Geometry: final body of the model. Coordinates: model frame, mm. A direction names the side the tool comes from. Round coordinates to 2 decimals unless told otherwise and drop trailing zeros. Answer in a Markdown table with one row per item.
Autodesk Inventor part; units mm, degrees
ref_plane "YZ Plane" through (0, 0, 0) normal (1, 0, 0) x (0, 1, 0)
ref_plane "XZ Plane" through (0, 0, 0) normal (0, 1, 0) x (-1, 0, 0)
ref_plane "XY Plane" through (0, 0, 0) normal (0, 0, 1) x (1, 0, 0)
sketch "Sketch1" plane through (0, 0, 0) normal (0, 0, 1) x (1, 0, 0)
  line L0 (-228.6, 101.6) -> (228.6, 101.6)
  line L1 (228.6, 101.6) -> (228.6, -101.6)
  line L2 (228.6, -101.6) -> (-228.6, -101.6)
  line L3 (-228.6, -101.6) -> (-228.6, 101.6)
  point P0 (0, 0)
  dimension "d0" = 457.2
  dimension "d1" = 203.2
  dimension "d2" = 228.6
  dimension "d3" = 101.6
extrude "Extrusion1" add sketch "Sketch1" along normal blind 6.35
sketch "Sketch2" plane through (0, 0, 6.35) normal (0, 0, 1) x (1, 0, 0)
  line L0 (-228.6, -101.6) -> (228.6, -101.6)
  line L1 (-196.85, -101.6) -> (-158.75, -101.6)
  line L2 (-158.75, -101.6) -> (-158.75, -63.5)
  line L3 (-158.75, -63.5) -> (-196.85, -63.5)
  line L4 (-196.85, -63.5) -> (-196.85, -101.6)
  line L5 (158.75, -101.6) -> (196.85, -101.6)
  line L6 (196.85, -101.6) -> (196.85, -63.5)
  line L7 (196.85, -63.5) -> (158.75, -63.5)
  line L8 (158.75, -63.5) -> (158.75, -101.6)
  line L9 (-228.6, 101.6) -> (-228.6, -101.6)
  line L10 (228.6, -101.6) -> (228.6, 101.6)
  point P0 (0, 0)
  dimension "d6" = 31.75
  dimension "d7" = 38.1
  dimension "d8" = 38.1
  dimension "d9" = 31.75
extrude "Extrusion2" cut sketch "Sketch2" against normal through all
chamfer "Chamfer1" distance 6.35 angle 45 4 edges at (196.85, -101.6, 3.175) (158.75, -101.6, 3.175) (-196.85, -101.6, 3.175) (-158.75, -101.6, 3.175)
sketch "Sketch3" plane through (0, 0, 0) normal (0, 0, -1) x (-1, 0, 0)
  circle A0 centre (-209.55, -88.9) radius 3.175
  circle A1 centre (-146.05, -88.9) radius 3.175
  circle A2 centre (146.05, -88.9) radius 3.175
  circle A3 centre (209.55, -88.9) radius 3.175
  line L0 (-152.4, -101.6) -> (152.4, -101.6)
  line L1 (-228.6, 101.6) -> (-228.6, -101.6)
  line L2 (228.6, -101.6) -> (228.6, 101.6)
  point P0 (0, 0)
  dimension "d15" = 12.7
  dimension "d16" = 6.35
  dimension "d17" = 19.05
  dimension "d18" = 63.5
  dimension "d19" = 63.5
  dimension "d20" = 19.05
extrude "Extrusion3" cut sketch "Sketch3" against normal blind 25.4
sketch "Sketch4" plane through (0, 0, 0) normal (0, 0, -1) x (-1, 0, 0)
  circle A0 centre (139.7, 76.2) radius 3.302
  circle A1 centre (165.1, 88.9) radius 3.302
  circle A2 centre (190.5, 76.2) radius 3.302
  circle A3 centre (215.9, 88.9) radius 3.302
  circle A4 centre (147.0661, 22.2869) radius 2.513
  circle A5 centre (177.1772, 22.2869) radius 2.513
  circle A6 centre (207.2882, 22.2869) radius 2.513
  circle A7 centre (207.2882, -28.5131) radius 2.513
  circle A8 centre (177.1772, -28.5131) radius 2.5956
  circle A9 centre (147.0661, -28.5131) radius 2.513
  circle A10 centre (-77.3373, 55.245) radius 1.5428
  circle A11 centre (52.0503, 55.245) radius 1.5428
  circle A12 centre (52.0503, -71.4248) radius 1.5428
  circle A13 centre (-77.3373, -71.4248) radius 1.5428
  arc A14 (-104.9183, -56.1295) -> (-107.5853, -58.7965) centre (-104.9183, -58.7965) ccw
  arc A15 (-102.2513, -58.7965) -> (-104.9183, -56.1295) centre (-104.9183, -58.7965) ccw
  arc A16 (-104.9183, -61.4635) -> (-102.2513, -58.7965) centre (-104.9183, -58.7965) ccw
  arc A17 (-107.5853, -58.7965) -> (-104.9183, -61.4635) centre (-104.9183, -58.7965) ccw
  arc A18 (77.3521, -56.1295) -> (74.6851, -58.7965) centre (77.3521, -58.7965) ccw
  arc A19 (74.6851, -58.7965) -> (77.3521, -61.4635) centre (77.3521, -58.7965) ccw
  arc A20 (77.3521, -61.4635) -> (80.0191, -58.7965) centre (77.3521, -58.7965) ccw
  arc A21 (80.0191, -58.7965) -> (77.3521, -56.1295) centre (77.3521, -58.7965) ccw
  arc A22 (80.0191, 45.5975) -> (77.3521, 48.2645) centre (77.3521, 45.5975) ccw
  arc A23 (77.3521, 48.2645) -> (74.6851, 45.5975) centre (77.3521, 45.5975) ccw
  arc A24 (74.6851, 45.5975) -> (77.3521, 42.9305) centre (77.3521, 45.5975) ccw
  arc A25 (77.3521, 42.9305) -> (80.0191, 45.5975) centre (77.3521, 45.5975) ccw
  arc A26 (-104.9183, 42.9305) -> (-102.2513, 45.5975) centre (-104.9183, 45.5975) ccw
  arc A27 (-107.5853, 45.5975) -> (-104.9183, 42.9305) centre (-104.9183, 45.5975) ccw
  arc A28 (-104.9183, 48.2645) -> (-107.5853, 45.5975) centre (-104.9183, 45.5975) ccw
  arc A29 (-102.2513, 45.5975) -> (-104.9183, 48.2645) centre (-104.9183, 45.5975) ccw
  circle A30 centre (-160.782, 71.882) radius 1.905
  circle A31 centre (-160.782, 24.13) radius 1.905
  circle A32 centre (-117.729, 24.1324) radius 1.905
  circle A33 centre (-117.729, 71.882) radius 1.905
  circle A34 centre (146.05, -88.9) radius 3.175
  circle A35 centre (-209.55, -88.9) radius 3.175
  circle A36 centre (-146.05, -88.9) radius 3.175
  circle A37 centre (209.55, -88.9) radius 3.175
  line L0 (158.75, -95.25) -> (152.4, -101.6)
  line L1 (158.75, -95.25) -> (158.75, -63.5)
  line L2 (158.75, -63.5) -> (196.85, -63.5)
  line L3 (196.85, -63.5) -> (196.85, -95.25)
  line L4 (203.2, -101.6) -> (196.85, -95.25)
  line L5 (203.2, -101.6) -> (228.6, -101.6)
  line L6 (228.6, -101.6) -> (228.6, 101.6)
  line L7 (228.6, 101.6) -> (-228.6, 101.6)
  line L8 (-228.6, 101.6) -> (-228.6, -101.6)
  line L9 (-228.6, -101.6) -> (-203.2, -101.6)
  line L10 (-196.85, -95.25) -> (-203.2, -101.6)
  line L11 (-196.85, -95.25) -> (-196.85, -63.5)
  line L12 (-196.85, -63.5) -> (-158.75, -63.5)
  line L13 (-158.75, -63.5) -> (-158.75, -95.25)
  line L14 (-152.4, -101.6) -> (-158.75, -95.25)
  line L15 (-152.4, -101.6) -> (152.4, -101.6)
  circle A38 centre (-177.8, 42.5448) radius 3.429
  circle A39 centre (-205.74, -14.6052) radius 3.429
  point P0 (0, 0)
extrude "Extrusion4" cut sketch "Sketch4" against normal through all contours A0 | A1 | A2 | A3 | A4 | A5 | A6 | A7 | A8 | A9 | A10 | A11 | A12 | A13 | A15 A16 A17 A14 | A21 A20 A19 A18 | A25 A24 A23 A22 | A27 A28 A29 A26 | A30 | A31 | A32 | A33 | A38 | A39
sketch "Sketch5" plane through (0, 0, 6.35) normal (0, 0, 1) x (1, 0, 0)
  line L0 (-90.717, 90.4998) -> (-91.3, 90.4141)
  line L1 (-91.3, 90.4141) -> (-91.3, 87.3859)
  line L2 (-91.3, 87.3859) -> (-90.717, 87.3002)
  arc A0 (-112.483, 87.3002) -> (-90.717, 87.3002) centre (-101.6, 88.9) ccw
  line L3 (-112.483, 87.3002) -> (-111.9, 87.3859)
  line L4 (-111.9, 87.3859) -> (-111.9, 90.4141)
  line L5 (-111.9, 90.4141) -> (-112.483, 90.4998)
  arc A1 (-103.0998, 99.7973) -> (-112.483, 90.4998) centre (-101.6, 88.9) ccw
  line L6 (-103.1, 101.3) -> (-103.0998, 99.7973)
  line L7 (-103.1, 101.3) -> (-100.1, 101.3)
  line L8 (-100.1002, 99.7973) -> (-100.1, 101.3)
  arc A2 (-90.717, 90.4998) -> (-100.1002, 99.7973) centre (-101.6, 88.9) ccw
  circle A3 centre (-101.6, 88.9) radius 17.9999
  circle A4 centre (-101.6, 88.9) radius 11
  point P0 (0, 0)
extrude "Extrusion5" cut sketch "Sketch5" against normal through all contours A4 L2 L1 L0 | L0 L1 L2 A0 L3 L4 L5 A1 A4 A2 | L5 L4 L3 A4
sketch "Sketch6" plane through (0, 0, 6.35) normal (0, 0, 1) x (1, 0, 0)
  circle A0 centre (-38.1565, 55.4101) radius 1.8832
  circle A1 centre (63.4435, 55.4101) radius 1.8832
  circle A2 centre (63.4435, -71.5899) radius 1.8832
  circle A3 centre (-38.1565, -71.5899) radius 1.8832
  point P0 (0, 0)
extrude "Extrusion6" cut sketch "Sketch6" against normal blind 25.4
equation "\"d9\" = d6"
equation "\"d19\" = d18"
equation "\"d20\" = d17"
properties part number "LexanPlate" material "Polycarbonate, Clear"
Item 1: Cut plane A-A (z = 3.75). Count the separate pieces of the cut face and the enclosed holes in it, then the cut area to 3 significant figures.
Answer:
| item | result |
|---|---|
| separate pieces | 1 |
| enclosed holes | 33 |
| area | 88,900 mm² |
Item 2: Pin query (flat end, axial travel): pin 1 Ø4 at (x, y) = (-190.5, 76.2) entering from -Z; pin 2 Ø8.5 at (x, y) = (-77.35, -58.8) entering from -Z; pin 3 Ø1.9 at (x, z) = (-179, 2) entering from -Y. Return the tip coordinate at first contact, or that it passes through.
Answer:
| item | result |
|---|---|
| pin 1 | passes through |
| pin 2 | stops at z = 0 |
| pin 3 | stops at y = -63.5 |
Item 3: Draft query along X for faces 1 (the face through (-101.8, 77.9, 3.2)), 2 (the face through (-3, 1, 0)). Return one class per face: pulls with the +X half, pulls with the -X half, needs draft (parallel to the pull), parting line crosses it, or undercut.
Answer:
| item | result |
|---|---|
| face 1 | undercut |
| face 2 | needs draft |
Item 4: Reachability of faces 3 (the face through (-93.788, 96.644, 3.219)), 4 (the face through (-3, 1, 6.35)) from +Z, -Z, +X, -X, +Y, -Y: full face, straight path, thin tool, end or side. Return the list, or none.
Answer:
| item | result |
|---|---|
| face 3 | +Z, -Z |
| face 4 | +Z, +X, -X, +Y, -Y |
Item 5: Line query: probe 1 along X at (y, z) = (72, 5); probe 2 along Y at (x, z) = (-215.9, 5); probe 3 along Y at (x, z) = (-100.5, 3.75). Output: solid intervals per line, ascending. Write a range as [from, to].
Answer:
| item | result |
|---|---|
| probe 1 | x = [-228.6, 115.83], [119.63, 158.88], [162.68, 228.6] |
| probe 2 | y = [-101.6, 85.6], [92.2, 101.6] |
| probe 3 | y = [-101.6, 77.96], [99.84, 101.6] |
